```python
from build123d import *

# Parameters (mm, degrees)
BOSS_EXTRU_1_DEPTH      = 2
BOSS_EXTRU_2_DEPTH      = 20
ESQUISSE4_R             = 7.5
ENL_V_MAT_EXTRU_1_DEPTH = 138.403473125


with BuildPart() as part:
    # Esquisse1 → Boss.-Extru.1 (new body)
    with BuildSketch(Plane(origin=(0, 0, 0), x_dir=(1, 0, 0), z_dir=(0, 1, 0))):
        with BuildLine():
            Line((-56.655462185, 33.12605042), (43.344537815, 33.12605042))
            ThreePointArc((43.344537815, 33.12605042), (58.900887001, 26.682399606), (65.344537815, 11.12605042))
            Line((65.344537815, 11.12605042), (65.344537815, -88.87394958))
            ThreePointArc((65.344537815, -88.87394958), (58.900887001, -104.430298766), (43.344537815, -110.87394958))
            Line((43.344537815, -110.87394958), (-56.655462185, -110.87394958))
            ThreePointArc((-56.655462185, -110.87394958), (-72.211811371, -104.430298766), (-78.655462185, -88.87394958))
            Line((-78.655462185, -88.87394958), (-78.655462185, 11.12605042))
            ThreePointArc((-78.655462185, 11.12605042), (-72.211811371, 26.682399606), (-56.655462185, 33.12605042))
        make_face()
    extrude(amount=BOSS_EXTRU_1_DEPTH)

    # Esquisse3 → Boss.-Extru.2 (add)
    with BuildSketch(Plane(origin=(0, 2, 0), x_dir=(1, 0, 0), z_dir=(0, 1, 0))):
        with BuildLine():
            Line((43.344537815, 31.12605042), (43.344537815, 29.12605042))
            ThreePointArc((43.344537815, 29.12605042), (56.072459876, 23.853972482), (61.344537815, 11.12605042))
            Line((61.344537815, 11.12605042), (63.344537815, 11.12605042))
            ThreePointArc((63.344537815, 11.12605042), (57.486673439, 25.268186044), (43.344537815, 31.12605042))
        make_face()
        with BuildLine():
            Line((43.344537815, -106.87394958), (43.344537815, -108.87394958))
            ThreePointArc((43.344537815, -108.87394958), (57.486673439, -103.016085204), (63.344537815, -88.87394958))
            Line((63.344537815, -88.87394958), (61.344537815, -88.87394958))
            ThreePointArc((61.344537815, -88.87394958), (56.072459876, -101.601871641), (43.344537815, -106.87394958))
        make_face()
        with BuildLine():
            Line((-76.655462185, -88.87394958), (-74.655462185, -88.87394958))
            ThreePointArc((-74.655462185, -88.87394958), (-69.383384246, -101.601871641), (-56.655462185, -106.87394958))
            Line((-56.655462185, -106.87394958), (-56.655462185, -108.87394958))
            ThreePointArc((-56.655462185, -108.87394958), (-70.797597809, -103.016085204), (-76.655462185, -88.87394958))
        make_face()
        with BuildLine():
            Line((-76.655462185, 11.12605042), (-74.655462185, 11.12605042))
            ThreePointArc((-74.655462185, 11.12605042), (-69.383384246, 23.853972482), (-56.655462185, 29.12605042))
            Line((-56.655462185, 29.12605042), (-56.655462185, 31.12605042))
            ThreePointArc((-56.655462185, 31.12605042), (-70.797597809, 25.268186044), (-76.655462185, 11.12605042))
        make_face()
    extrude(amount=BOSS_EXTRU_2_DEPTH)

    # Esquisse4 → Enlèv. mat.-Extru.1 (cut, through all)
    with BuildSketch(Plane(origin=(0, 2, 0), x_dir=(1, 0, 0), z_dir=(0, 1, 0))):
        with Locations(Location((-6.655462185, -38.87394958, 0), (0, 0, 270))):
            Circle(ESQUISSE4_R)
    extrude(amount=-ENL_V_MAT_EXTRU_1_DEPTH, mode=Mode.SUBTRACT)


solid = part.part
```
For this review, take the finished solid that the model builds, in its own axes (mm). A direction names the side the tool comes from. Round coordinates to 2 decimals unless told otherwise and drop trailing zeros. Write each loop counter-clockwise with the first axis right and the second up, starting at its lowest first coordinate (ties: lowest second). Pieces come first, ordered by that corner, then holes. Notation, with made-up numbers: (15, 59.5) - (50, 59.5) arc R28 ccw to (50, 85.5) - close; hole circle Ø6 at (-29.75, -6.5). An arc over 180 degrees is marked (long way). Answer as CSV lines item,"result". Start each with the question number.
(1) Add section A-A, the plane y = 17. State the section outline as (x, z) points.
(2) Machinability: for faces 4 (the cylindrical face through (-70.64, 11.86, 103.17)), 5 (the cylindrical face through (57.641, 11.86, -25.112)), 6 (the flat face through (56, 22, 102)), 7 (the cylindrical face through (-70.641, 11.86, -25.423)), 8 (the cylindrical face through (55.932, 11.86, -23.993)), which of the approach directions +Z, -Z, +X, -X, +Y, -Y give a long, thin tool a straight path to every point of the face, cutting with its end or side? Answer none if there is none.
(3) For pin 1 (1.5 mm diameter, centred on x = 11, z = -14, fed in from +Y); pin 2 (1.6 mm diameter, centred on y = 13.5, z = 107.5, fed in from -X); pin 3 (0.6 mm diameter, centred on x = 62, y = 8.5, fed in from -Z); pin 4 (10 mm diameter, centred on x = 14.5, z = -10, fed in from -Y), all flat-tipped, find the tip position at first contact; note any pin that passes through.
(4) For line 1 (Y direction, x = 47, z = 0.5); line 2 (X direction, y = 3.25, z = -17); line 3 (X direction, y = 20.5, z = -16), list the stretches that pass through material, from the lowest coordinate up.
(5) Add section C-C, the plane x = 21. State the section outline as (y, z) points.
(6) Mouldability with a two-part tool opening along X and no side actions: class faces 1 (the cylindrical face through (-72.04, 0.99, 104.6)), 2 (the cylindrical face through (57.3, 11.9, 103.2)), 3 (the cylindrical face through (-13.977, 1.014, 37.248)) as +X half, -X half, draft (parallel to the pull), parting line (faces both ways), or undercut.
(7) Add section D-D, the plane z = 23. State the section outline as (x, y) points, plus the area to 3 significant figures.
(8) Add section B-B, the plane z = 43.5. State the section outline as (x, y) points.
From the geometry:
1,outline,"(-76.66, -11.13) arc R20 ccw to (-56.66, -31.13) - (-56.66, -29.13) arc R18 cw to (-74.66, -11.13) - close; (-76.66, 88.87) - (-74.66, 88.87) arc R18 cw to (-56.66, 106.87) - (-56.66, 108.87) arc R20 ccw to start; (43.34, -31.13) arc R20 ccw to (63.34, -11.13) - (61.34, -11.13) arc R18 cw to (43.34, -29.13) - close; (43.34, 106.87) arc R18 cw to (61.34, 88.87) - (63.34, 88.87) arc R20 ccw to (43.34, 108.87) - close"
2,face 4,"+Z, -X, +Y"
2,face 5,"-Z, +X, +Y"
2,face 6,"+Z, -Z, +X, -X, +Y"
2,face 7,"-Z, -X, +Y"
2,face 8,"+Y"
3,pin 1,"stops at y = 2"
3,pin 2,"stops at x = -65.72"
3,pin 3,"stops at z = -19.07"
3,pin 4,"stops at y = 0"
4,line 1,"y = 0 to 2"
4,line 2,"x = -75.77 to -73.67, 60.36 to 62.46"
4,line 3,"x = -76.05 to -73.98, 60.67 to 62.74"
5,outline,"(0, -33.13) - (2, -33.13) - (2, 110.87) - (0, 110.87) - close"
6,face 1,"-X half"
6,face 2,"+X half"
6,face 3,"undercut"
7,outline,"(-78.66, 0) - (65.34, 0) - (65.34, 2) - (-78.66, 2) - close"
7,area,"288 mm²"
8,outline,"(-78.66, 0) - (-12.56, 0) - (-12.56, 2) - (-78.66, 2) - close; (-0.75, 0) - (65.34, 0) - (65.34, 2) - (-0.75, 2) - close"
